Solid Edge part; units mm, degrees
sketch "Sketch1" plane through (0, 0, 0) normal (0, 0, 1) x (1, 0, 0)
  line L0 (0, 0) -> (-170.02, 0)
  line L1 (-170.02, 0) -> (-170.02, -85)
  line L2 (-170.02, -85) -> (0, -85)
  line L3 (0, -85) -> (0, 0)
extrude "Protrusion1" add sketch "Sketch1" against normal blind 20.4
sketch "Sketch2" plane through (-85.01, -42.5, 0) normal (0, 0, 1) x (0, 1, 0)
  circle A0 centre (-9, 42.49) radius 6.7
  circle A1 centre (-9, -42.51) radius 6.7
  circle A2 centre (-7, -120.01) radius 57.5
  circle A3 centre (-7, 119.99) radius 57.5
extrude "ExtrudedCutout_1" cut sketch "Sketch2" against normal blind 20.5
chamfer "Chamfer_2" distance 2 angle 65 1 edges at (-10.2327, -85, -10.2) measured on face at (-136.3402, -85, -16.796)
chamfer "Chamfer_3" distance 2 angle 65 1 edges at (-159.7673, -85, -10.2) measured on face at (-136.6535, -85, -16.796)
chamfer "Chamfer_4" distance 2 angle 65 1 edges at (-170.02, 0, -10.2) measured on face at (-26.6365, 0, -16.796)
chamfer "Chamfer_5" distance 2 angle 65 1 edges at (0, 0, -10.2) measured on face at (-26.3231, 0, -16.796)
For this review, take the finished solid that the model builds, in its own axes (mm). Give positions to 0.01 mm unless a question says otherwise; leave off trailing zeros. Write each loop counter-clockwise with the first axis right and the second up, starting at its lowest first coordinate (ties: lowest second). Pieces come first, ordered by that corner, then holes.
Item 1: Insertion check: P1, Ø17.5, axis at x = -127.5, y = -51.5, coming from the -Z side; P2, Ø1, axis at y = -11, z = -15.5, coming from the +X side; P3, Ø2, axis at y = -18.5, z = -3, coming from the -X side. Each pin has a flat end and moves straight along its axis. Give the tip position at first contact, or say it passes through.
Item 2: Take a section at C-C (z = -12.5). Give the boundary of the cut face in (x, y).
Item 3: The part is to be moulded in two halves that separate along X. For faces 1 (the face through (-21.83, -40.76, -10.06)), 2 (the face through (-168.96, -2.02, -10.06)), 3 (the face through (-132.028, -56.438, -10.057)), say which applies: +X half, -X half, draft (parallel to the pull), parting line (faces both ways), or undercut.
Item 4: Take a section at A-A (x = -127.5). Give the boundary of the cut face in (y, z).
Item 5: Take a section at B-B (y = -50). Give the boundary of the cut face in (x, z).
Item 6: Wall thickness on probe 1 along X at (y, z) = (-51.5, -13.5); probe 2 along Y at (x, z) = (-127.5, -8.25); probe 3 along X at (y, z) = (-48.5, -14): over which ranges is each line inside the solid? List them lowest first.
Item 7: Take a section at D-D (x = -38.5). Give the boundary of the cut face in (y, z).
Established:
1. P1: stops at z = -20.4
1. P2: stops at x = -7.25
1. P3: stops at x = -157.23
2. outline: (-169.87, -3.98) arc R57.5 cw to (-158.53, -83.36) - (-157.77, -85) - (-12.23, -85) - (-11.47, -83.36) arc R57.5 cw to (-0.14, -3.99) - (-2, 0) - (-168.02, 0) - close; hole circle Ø13.4 at (-127.5, -51.5); hole circle Ø13.4 at (-42.5, -51.5)
3. face 1: +X half
3. face 2: -X half
3. face 3: undercut
4. outline: (-85, -20.4) - (-58.2, -20.4) - (-58.2, 0) - (-85, 0) - close; (-44.8, -20.4) - (0, -20.4) - (0, 0) - (-44.8, 0) - close
5. outline: (-147.5, -20.4) - (-134.03, -20.4) - (-134.03, 0) - (-147.5, 0) - close; (-120.97, -20.4) - (-49.03, -20.4) - (-49.03, 0) - (-120.97, 0) - close; (-35.97, -20.4) - (-22.5, -20.4) - (-22.5, 0) - (-35.97, 0) - close
6. probe 1: x = -147.53 to -134.2, -120.8 to -49.2, -35.8 to -22.47
6. probe 2: y = -85 to -58.2, -44.8 to 0
6. probe 3: x = -147.51 to -133.49, -121.51 to -48.49, -36.51 to -22.49
7. outline: (-85, -20.4) - (-56.87, -20.4) - (-56.87, 0) - (-85, 0) - close; (-46.13, -20.4) - (0, -20.4) - (0, 0) - (-46.13, 0) - close
